Can you work these out from the model? Positions are in its coordinate system, mm. A direction names the side the tool comes from. Round coordinates to 2 decimals unless told otherwise and drop trailing zeros. Loops run counter-clockwise (first coordinate to the right, second up) from the corner with the lowest first, then second, coordinate; pieces in that order, holes last. Notation, with made-up numbers: (87, 64.5) - (117, 64.5) arc R8 ccw to (117, 74.5) - close; hole circle Ø7 at (72, 26). An arc over 180 degrees is marked (long way). Answer as CSV lines item,"result".
Autodesk Inventor part; units mm, degrees
ref_plane "YZ Plane" through (0, 0, 0) normal (1, 0, 0) x (0, 1, 0)
ref_plane "XZ Plane" through (0, 0, 0) normal (0, 1, 0) x (-1, 0, 0)
ref_plane "XY Plane" through (0, 0, 0) normal (0, 0, 1) x (1, 0, 0)
sketch "Sketch1" plane through (0, 0, 0) normal (0, 0, 1) x (1, 0, 0)
  line L0 (0, -8.2641) -> (0, 19.7359)
  line L1 (-162.5659, 0) -> (21.6343, 0) construction
  line L2 (-107.95, 8.89) -> (-107.95, -8.89) construction
  line L3 (-107.95, 8.89) -> (-90.3815, 8.89) construction
  line L4 (-90.3815, 8.89) -> (-90.3815, 7.3025) construction
  line L5 (-90.3815, 7.3025) -> (-91.504, 6.18) construction
  line L6 (-91.504, 6.18) -> (-92.9409, 7.6168) construction
  line L7 (-92.9409, 7.6168) -> (-95.186, 5.3717) construction
  line L8 (-95.186, 5.3717) -> (-93.7491, 3.9349) construction
  line L9 (-93.7491, 3.9349) -> (-97.684, 0) construction
  line L10 (-97.176, 0) -> (-84.8354, 12.3406) construction
  line L11 (-94.0634, 6.4943) -> (-92.3726, 4.8034) construction
  circle A0 centre (-93.218, 5.6489) radius 1.3081 construction
  line L12 (-90.3815, -8.89) -> (-90.3815, -7.3025) construction
  line L13 (-90.3815, -7.3025) -> (-91.504, -6.18) construction
  line L14 (-91.504, -6.18) -> (-92.9409, -7.6168) construction
  line L15 (-92.9409, -7.6168) -> (-95.186, -5.3717) construction
  line L16 (-95.186, -5.3717) -> (-93.7491, -3.9349) construction
  line L17 (-93.7491, -3.9349) -> (-97.684, 0) construction
  line L18 (-107.95, -8.89) -> (-90.3815, -8.89) construction
  line L19 (-89.6195, 8.89) -> (-89.6195, 7.5565)
  line L20 (-89.6195, 7.5565) -> (-97.176, 0)
  line L21 (-89.6195, 8.89) -> (-77.7875, 8.89)
  line L22 (-77.7875, 8.89) -> (-77.7875, -8.89)
  line L23 (-89.6195, -8.89) -> (-89.6195, -7.5565)
  line L24 (-89.6195, -7.5565) -> (-97.176, 0)
  line L25 (-89.6195, -8.89) -> (-77.7875, -8.89)
  point P0 (0, 0)
  point P1 (0, 0)
  point P2 (0, 0)
  dimension "d23" = 1.5875
  dimension "d24" = 2.032
  dimension "d25" = 45
  dimension "d26" = 0.508
  dimension "d27" = 3.175
  dimension "d28" = 2.6162
  dimension "d29" = 186.436
  dimension "d30" = 215.9
  dimension "d31" = 17.78
  dimension "d32" = 1.5875
  dimension "d33" = 0.762
  dimension "d34" = 155.575
  dimension "d35" = 17.78
revolve "Revolution1" add sketch "Sketch1" angle 360 about axis through (0, -8.2641, 0) along (0, 1, 0)
properties part number "3DPRINT,INNER-V" material "Nylon 6/6"
Q1. If I drill on line 1 along X through (y, z) = (-6.25, -58); line 2 along Z through (x, y) = (-30, 2); line 3 along X through (y, z) = (0, 12), over which ranges is the centre line in solid material (lowest first)? Write a range as [from, to].
Checks:
line 1,"[-70.03, -51.84], [51.84, 70.03]"
line 2,"[-90.32, -71.77], [71.77, 90.32]"
line 3,"[-96.43, -76.86], [76.86, 96.43]"
Q2. Imagine slicing it at C-C (y = 4.25). Write out the boundary of the cut face in (x, z) (1 decimal).
Checks:
outline,"circle Ø185.9 at (0, 0); hole circle Ø155.6 at (0, 0)"
Q3. We'd pull the mould along Z, two halves only. Please class faces 3 (the flat face through (27, 8.89, 73.4)), 4 (the cylindrical face through (61.73, -0.12, 47.33)), 5 (the cylindrical face through (66.05, 8.21, -60.57)): pulls with the +Z half, pulls with the -Z half, needs draft (parallel to the pull), parting line crosses it, or undercut.
Checks:
face 3,"needs draft"
face 4,"undercut"
face 5,"parting line crosses it"
Q4. I'm going to push flat-ended pins straight in: pin 1 Ø8 at (y, z) = (-5.5, 9) entering from -X; pin 2 Ø2 at (y, z) = (-3, 37) entering from -X; pin 3 Ø6 at (x, y) = (-41, 6) entering from +Z. Where does each tip first touch, or does it pass through?
Checks:
pin 1,"x = -95.27"
pin 2,"x = -87.77"
pin 3,"z = 85.08"
Q5. On a 3-axis mill with a long thin cutter (end or side, diameter ignored), from which of +Z, -Z, +X, -X, +Y, -Y can I reach the whole of each face in a straight line? I mean faces 1 (the flat face through (27, -8.89, 73.4)), 2 (the cylindrical face through (66.05, -8.21, 60.57)). Say none if no direction works.
Checks:
face 1,"+Z, -Z, +X, -X, -Y"
face 2,"-Y"
Q6. Imagine slicing it at A-A (x = 0). Write out the boundary of the cut face in (y, z), then the cut area to 3 significant figures.
Checks:
outline,"(-8.89, -89.62) - (-7.56, -89.62) - (0, -97.18) - (7.56, -89.62) - (8.89, -89.62) - (8.89, -77.79) - (-8.89, -77.79) - close; (-8.89, 77.79) - (8.89, 77.79) - (8.89, 89.62) - (7.56, 89.62) - (0, 97.18) - (-7.56, 89.62) - (-8.89, 89.62) - close"
area,"535 mm²"
Q7. Imagine slicing it at B-B (z = 0). Write out the boundary of the cut face in (x, y), then the cut area to 3 significant figures.
Checks:
outline,"(-97.18, 0) - (-89.62, -7.56) - (-89.62, -8.89) - (-77.79, -8.89) - (-77.79, 8.89) - (-89.62, 8.89) - (-89.62, 7.56) - close; (77.79, -8.89) - (89.62, -8.89) - (89.62, -7.56) - (97.18, 0) - (89.62, 7.56) - (89.62, 8.89) - (77.79, 8.89) - close"
area,"535 mm²"
